```python
from build123d import *

# Parameters (mm, degrees)
SKETCH1_R           = 2
BOSS_EXTRUDE1_DEPTH = 5
SKETCH2_R           = 2
SKETCH2_R_2         = 1.5875
BOSS_EXTRUDE2_DEPTH = 5
SKETCH3_R           = 2
SKETCH3_R_2         = 1.5875
BOSS_EXTRUDE3_DEPTH = 5


with BuildPart() as part:
    # Sketch1 → Boss-Extrude1 (new body)
    with BuildSketch(Plane.XY.offset(63)):
        with BuildLine():
            Line((8.181928414, -16.605718064), (17.802171103, -33.691169181))
            ThreePointArc((17.802171103, -33.691169181), (18.572370652, -35.426303597), (19.000782012, -37.275725803))
            ThreePointArc((19.000782012, -37.275725803), (24.928229029, -40.232462465), (25.473776059, -33.631000637))
            ThreePointArc((25.473776059, -33.631000637), (24.114589128, -32.30566684), (23.030358602, -30.747352701))
            Line((23.030358602, -30.747352701), (13.410115914, -13.661901584))
            ThreePointArc((13.410115914, -13.661901584), (12.639916365, -11.926767167), (12.211505005, -10.077344962))
            ThreePointArc((12.211505005, -10.077344962), (6.284057988, -7.1206083), (5.738510958, -13.722070128))
            ThreePointArc((5.738510958, -13.722070128), (7.097697889, -15.047403925), (8.181928414, -16.605718064))
        make_face()
        with Locations(Location((8.246602308, -10.606066633, 0), (0, 0, 180))):
            Circle(SKETCH1_R, mode=Mode.SUBTRACT)
        with Locations(Location((22.965684708, -36.747004132, 0), (0, 0, 180))):
            Circle(SKETCH1_R, mode=Mode.SUBTRACT)
    extrude(amount=-BOSS_EXTRUDE1_DEPTH)

    # Sketch2 → Boss-Extrude2 (add, through all)
    with BuildSketch(Plane(origin=(0, 0, 58), x_dir=(-1, 0, 0), z_dir=(0, 0, -1))):
        with Locations((-22.965684708, -36.747004132)):
            Circle(SKETCH2_R)
        with Locations((-22.965684708, -36.747004132)):
            Circle(SKETCH2_R_2, mode=Mode.SUBTRACT)
    extrude(amount=-BOSS_EXTRUDE2_DEPTH)

    # Sketch3 → Boss-Extrude3 (add, through all)
    with BuildSketch(Plane(origin=(0, 0, 58), x_dir=(-1, 0, 0), z_dir=(0, 0, -1))):
        with Locations((-8.246602308, -10.606066633)):
            Circle(SKETCH3_R)
        with Locations((-8.246602308, -10.606066633)):
            Circle(SKETCH3_R_2, mode=Mode.SUBTRACT)
    extrude(amount=-BOSS_EXTRUDE3_DEPTH)


solid = part.part
```
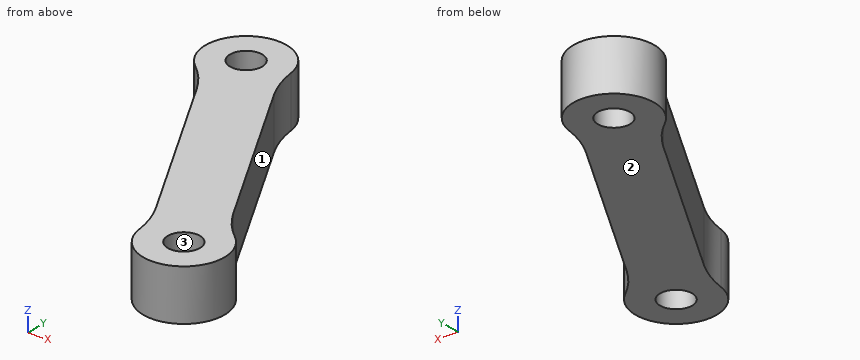
Model file for the job. Use its own axes, mm. Face numbers are marked on the shaded views. Round coordinates to 2 decimals unless told otherwise and drop trailing zeros. Write each loop counter-clockwise with the first axis right and the second up, starting at its lowest first coordinate (ties: lowest second). Pieces come first, ordered by that corner, then holes. Notation, with made-up numbers: (8.5, 52.25) - (15.5, 52.25) arc R22 cw to (15.5, 67.25) - close; hole circle Ø5 at (86, 29.25). An arc over 180 degrees is marked (long way). One line per item, written item: value.
(1) Cut at B-B, the plane z = 60.55. Give the cut face in (x, y) (1 decimal), plus the area to 3 significant figures.
Values follow:
outline: (5.7, -13.7) arc R10 cw to (8.2, -16.6) - (17.8, -33.7) arc R10 cw to (19, -37.3) arc R4 ccw (long way) to (25.5, -33.6) arc R10 cw to (23, -30.7) - (13.4, -13.7) arc R10 cw to (12.2, -10.1) arc R4 ccw (long way) to start; hole circle Ø3.2 at (8.2, -10.6); hole circle Ø3.2 at (23, -36.7)
area: 223 mm²
(2) Cut at A-A, the plane y = -38. Give the cut face in (x, z).
Values follow:
outline: (19.17, 58) - (21.99, 58) - (21.99, 63) - (19.17, 63) - close; (23.94, 58) - (26.76, 58) - (26.76, 63) - (23.94, 63) - close
(3) Cut at D-D, the plane y = -14.5. Give the cut face in (x, z), plus the area to 3 significant figures.
Values follow:
outline: (6.6, 58) - (13.88, 58) - (13.88, 63) - (6.6, 63) - close
area: 36.4 mm²
(4) Two-plate mould, pull along Y, no slides. Class the marked faces 1, 2 and 3: pulls with the +Y half, pulls with the -Y half, needs draft (parallel to the pull), parting line crosses it, or undercut.
Values follow:
face 1: pulls with the +Y half
face 2: needs draft
face 3: undercut
(5) Cut at C-C, the plane x = 20.25. Give the cut face in (y, z).
Values follow:
outline: (-39.68, 58) - (-25.81, 58) - (-25.81, 63) - (-39.68, 63) - close
(6) Drop flat-ended pins along their axis: P1, Ø3, axis at y = -20, z = 61, coming from the +X side; P2, Ø3, axis at y = -22, z = 62.5, coming from the +X side. Give the stop position or say it passes through.
Values follow:
P1: stops at x = 17.82
P2: stops at x = 18.95
(7) Wall check: probe 1 along Y at (x, z) = (22.75, 60.2); probe 2 along X at (y, z) = (-12, 62.1); probe 3 along Y at (x, z) = (22.5, 59.3). Give the ranges that are in metal, low to high.
Values follow:
probe 1: y = -40.74 to -38.32, -35.17 to -30.25
probe 2: x = 4.5 to 7.49, 9.01 to 12.66
probe 3: y = -40.72 to -38.26, -35.23 to -29.81
